Input: part model. Units: mm. Frame: model coordinates. Round coordinates to 2 decimals unless told otherwise and drop trailing zeros. Write each loop counter-clockwise with the first axis right and the second up, starting at its lowest first coordinate (ties: lowest second). Pieces come first, ordered by that corner, then holes. Notation, with made-up numbers: M 29,-36 L 86,-36 A26 ccw 86,-19 Z; hole C 88,35.5 d5. An arc over 180 degrees is marked long. Write each question's results on one line, items separated by ' | '. Start each with the question number.
Autodesk Inventor part; units mm, degrees
ref_plane "YZ Plane" through (0, 0, 0) normal (1, 0, 0) x (0, 1, 0)
ref_plane "XZ Plane" through (0, 0, 0) normal (0, 1, 0) x (-1, 0, 0)
ref_plane "XY Plane" through (0, 0, 0) normal (0, 0, 1) x (1, 0, 0)
sketch "Sketch1" plane through (0, 0, 0) normal (0, 0, 1) x (1, 0, 0)
  line L0 (-102.5157, 69.2842) -> (97.4843, 69.2842)
  line L1 (97.4843, 69.2842) -> (97.4843, -80.7158)
  line L2 (97.4843, -80.7158) -> (-102.5157, -80.7158)
  line L3 (-102.5157, -80.7158) -> (-102.5157, 69.2842)
  point P0 (0, 0)
extrude "Extrusion1" add sketch "Sketch1" along normal blind 3
sketch "Sketch3" plane through (0, 0, 3) normal (0, 0, 1) x (1, 0, 0)
  point P0 (0, 0)
sketch "Sketch4" plane through (0, 0, 3) normal (0, 0, 1) x (1, 0, 0)
  line L0 (97.4843, 69.2842) -> (-102.5157, 69.2842)
  line L1 (-102.5157, 69.2842) -> (-99.5157, 69.2842)
  line L2 (-99.5157, 69.2842) -> (-99.5157, 19.2842)
  line L3 (-99.5157, 19.2842) -> (-102.5157, 19.2842)
  line L4 (-102.5157, 19.2842) -> (-102.5157, 69.2842)
  point P0 (0, 0)
extrude "Extrusion2" cut sketch "Sketch4" against normal blind 3
sketch "Sketch5" plane through (0, 0, 3) normal (0, 0, 1) x (1, 0, 0)
  line L0 (97.4843, -80.7158) -> (94.4843, -80.7158)
  line L1 (94.4843, -80.7158) -> (94.4843, -30.7158)
  line L2 (94.4843, -30.7158) -> (97.4843, -30.7158)
  line L3 (97.4843, -30.7158) -> (97.4843, -80.7158)
  point P0 (0, 0)
  point P1 (-102.5157, -80.7158)
  dimension "d17" = 3
  dimension "d18" = 50
extrude "Extrusion3" cut sketch "Sketch5" against normal blind 3
sketch "Sketch6" plane through (0, 0, 3) normal (0, 0, 1) x (1, 0, 0)
  line L0 (97.4843, -30.7158) -> (97.4843, 69.2842)
  line L1 (97.4843, 69.2842) -> (94.4843, 69.2842)
  line L2 (94.4843, 69.2842) -> (94.4843, 19.2842)
  line L3 (94.4843, 19.2842) -> (97.4843, 19.2842)
  line L4 (97.4843, 19.2842) -> (97.4843, 69.2842)
  point P0 (0, 0)
  dimension "d21" = 50
  dimension "d22" = 3
extrude "Extrusion4" cut sketch "Sketch6" against normal blind 3
sketch "Sketch7" plane through (0, 0, 3) normal (0, 0, 1) x (1, 0, 0)
  line L0 (-102.5157, 19.2842) -> (-102.5157, -80.7158)
  line L1 (-102.5157, -80.7158) -> (-99.5157, -80.7158)
  line L2 (-99.5157, -80.7158) -> (-99.5157, -30.7158)
  line L3 (-99.5157, -30.7158) -> (-102.5157, -30.7158)
  line L4 (-102.5157, -30.7158) -> (-102.5157, -80.7158)
  point P0 (0, 0)
  dimension "d25" = 50
  dimension "d26" = 3
extrude "Extrusion5" cut sketch "Sketch7" against normal blind 3
sketch "Sketch8" plane through (0, 0, 3) normal (0, 0, 1) x (1, 0, 0)
  line L0 (-102.5157, -30.7158) -> (-102.5157, 19.2842)
  line L1 (97.4843, -30.7158) -> (94.4843, -30.7158)
  line L2 (94.4843, -80.7158) -> (-99.5157, -80.7158)
  line L3 (-10.0157, -50.7158) -> (4.9843, -50.7158)
  line L4 (4.9843, -50.7158) -> (4.9843, -80.7158)
  line L5 (4.9843, -80.7158) -> (-10.0157, -80.7158)
  line L6 (-10.0157, -80.7158) -> (-10.0157, -50.7158)
  point P0 (0, 0)
  dimension "d32" = 15
  dimension "d33" = 30
extrude "Extrusion6" cut sketch "Sketch8" against normal blind 3
sketch "Sketch9" plane through (-10.0157, -50.7158, 3) normal (0, -1, 0) x (1, 0, 0)
  line L0 (0, 0) -> (15, 0)
  line L1 (15, -3) -> (0, -3)
  line L2 (0, 0) -> (15, 0)
  line L3 (15, 0) -> (15, -3)
  line L4 (15, -3) -> (0, -3)
  line L5 (0, -3) -> (0, 0)
  point P0 (10.0157, -3)
extrude "Extrusion7" add sketch "Sketch9" along normal blind 30
sketch "Sketch10" plane through (0, 0, 0) normal (0, 0, -1) x (-1, 0, 0)
  line L0 (-94.4843, 69.2842) -> (99.5157, 69.2842)
  line L1 (99.5157, -80.7158) -> (-94.4843, -80.7158)
  line L2 (-97.4843, 19.2842) -> (-97.4843, -30.7158)
  line L3 (102.5157, 19.2842) -> (102.5157, -30.7158)
  line L4 (2.5157, 69.2842) -> (102.5157, 69.2842)
  circle A0 centre (-12.4843, 59.2842) radius 5
  circle A1 centre (17.5157, 59.2842) radius 5
  circle A2 centre (-12.4843, -70.7158) radius 5
  circle A3 centre (17.5157, -70.7158) radius 5
  point P0 (0, 0)
extrude "Extrusion8" cut sketch "Sketch10" against normal blind 24.75
properties part number "Level1"
1. Cut plane C-C on y = 46.5. Output: boundary loops of the cut face in (x, z).
2. Line query: L1, parallel to X at y = 59.5, z = 1.25; L2, parallel to X at y = 58.5, z = 1.3; L3, parallel to X at y = 49, z = 1. Output: solid intervals per line, ascending. Write a range as from..to.
3. Cut plane A-A on x = 14.5. Output: boundary loops of the cut face in (y, z).
4. Cut plane B-B on z = 0.7. Output: boundary loops of the cut face in (x, y), and give its area (3 significant figures).
5. Contact query for flat-ended pins moving along their axis: P1, Ø1.5, axis at y = 43, z = 1.5, coming from the -X side; P2, Ø1.5, axis at x = -101, z = 1, coming from the -Y side; P3, Ø6, axis at x = -17.52, y = 59.28, coming from the +Z side; P4, Ø1.5, axis at x = 96, z = 1, coming from the +Y side. Output: stop coordinate, or through.
6. Draft query along Y for faces 1 (the face through (-4, -5, 3)), 2 (the face through (-12.52, 59.5, 1.48)). Return one class per face: +Y half, -Y half, draft (parallel to the pull), parting line (faces both ways), or undercut.
Answers follow:
1) outline: M -99.52,0 L 94.48,0 L 94.48,3 L -99.52,3 Z
2) L1: x = -99.52..-22.51, -12.52..7.49, 17.48..94.48 | L2: x = -99.52..-22.45, -12.58..7.55, 17.42..94.48 | L3: x = -99.52..94.48
3) outline: M -80.72,0 L -75.29,0 L -75.29,3 L -80.72,3 Z; M -66.14,0 L 54.71,0 L 54.71,3 L -66.14,3 Z; M 63.86,0 L 69.28,0 L 69.28,3 L 63.86,3 Z
4) outline: M -102.52,-30.72 L -99.52,-30.72 L -99.52,-80.72 L 94.48,-80.72 L 94.48,-30.72 L 97.48,-30.72 L 97.48,19.28 L 94.48,19.28 L 94.48,69.28 L -99.52,69.28 L -99.52,19.28 L -102.52,19.28 Z; hole C -17.52,-70.72 d10; hole C -17.52,59.28 d10; hole C 12.48,-70.72 d10; hole C 12.48,59.28 d10 | area: 29,100 mm2
5) P1: stops at x = -99.52 | P2: stops at y = -30.72 | P3: passes through | P4: stops at y = 19.28
6) face 1: draft | face 2: undercut
